Read the model definition and answer for the solid it produces. Units are mm, in the model's axes. A direction names the side the tool comes from. Give positions to 0.01 mm unless a question says otherwise; leave off trailing zeros. Order: outer loops, then holes, each group sorted by start corner. A loop starts at its lowest first (then second) coordinate and runs counter-clockwise, first axis right, second up. Notation, with made-up numbers: M 31.5,33 L 85.5,33 A15 cw 85.5,62 Z; hole C -2.75,63 d3. An arc over 180 degrees is marked long. One line per item, written item: value.
from build123d import *

# Parameters (mm, degrees)
SKETCH1_W           = 12.7
SKETCH1_H           = 50.8
BOSS_EXTRUDE1_DEPTH = 15.113
BOSS_EXTRUDE2_START = 15.113
SKETCH1_3_R         = 25.4
SKETCH1_3_R_2       = 11.303
SKETCH1_3_R_3       = 5.588
SKETCH1_3_W         = 12.7
SKETCH1_3_H         = 50.8
BOSS_EXTRUDE2_DEPTH = 8.636
BOSS_EXTRUDE3_START = 23.749
SKETCH1_4_R         = 5.588
SKETCH1_4_W         = 12.7
SKETCH1_4_H         = 50.8
BOSS_EXTRUDE3_DEPTH = 6.477
SKETCH2_R           = 9.525
CUT_EXTRUDE1_DEPTH  = 130.132211086
SKETCH3_R           = 17.526
CUT_EXTRUDE2_DEPTH  = 2.3876


with BuildPart() as part:
    # Sketch1 → Boss-Extrude1 (new body)
    with BuildSketch(Plane(origin=(0, 0, 0), x_dir=(0, 0, -1), z_dir=(1, 0, 0))):
        with Locations((6.35, 25.4)):
            Rectangle(SKETCH1_W, SKETCH1_H)
    boss_extrude1 = extrude(amount=BOSS_EXTRUDE1_DEPTH)

    # Sketch1_3 → Boss-Extrude2 (add)
    with BuildSketch(Plane(origin=(0, 0, 0), x_dir=(0, 0, -1), z_dir=(1, 0, 0)).offset(BOSS_EXTRUDE2_START)):
        with BuildLine():
            Line((22.86, 50.8), (43.688, 0))
            Line((43.688, 0), (89.408, 0))
            ThreePointArc((89.408, 0), (64.008, 25.4), (89.408, 50.8))
            Line((89.408, 50.8), (22.86, 50.8))
        make_face()
        with Locations((89.408, 25.4)):
            Circle(SKETCH1_3_R)
        with Locations((89.408, 25.4)):
            Circle(SKETCH1_3_R_2, mode=Mode.SUBTRACT)
        Polygon((12.7, 50.8), (12.7, 0), (43.688, 0), (22.86, 50.8), align=None)
        with Locations((28.956, 17.78)):
            Circle(SKETCH1_3_R_3, mode=Mode.SUBTRACT)
        with Locations((6.35, 25.4)):
            Rectangle(SKETCH1_3_W, SKETCH1_3_H)
    boss_extrude2 = extrude(amount=BOSS_EXTRUDE2_DEPTH)

    # Sketch1_4 → Boss-Extrude3 (add)
    with BuildSketch(Plane(origin=(0, 0, 0), x_dir=(0, 0, -1), z_dir=(1, 0, 0)).offset(BOSS_EXTRUDE3_START)):
        Polygon((12.7, 50.8), (12.7, 0), (43.688, 0), (22.86, 50.8), align=None)
        with Locations((28.956, 17.78)):
            Circle(SKETCH1_4_R, mode=Mode.SUBTRACT)
        with Locations((6.35, 25.4)):
            Rectangle(SKETCH1_4_W, SKETCH1_4_H)
    boss_extrude3 = extrude(amount=BOSS_EXTRUDE3_DEPTH)

    # Mirror1: Boss-Extrude1, Boss-Extrude2, Boss-Extrude3 across plane
    add(boss_extrude1.mirror(Plane(origin=(0, 0, 0), x_dir=(0, 0, 1), z_dir=(1, 0, 0))))
    add(boss_extrude2.mirror(Plane(origin=(0, 0, 0), x_dir=(0, 0, 1), z_dir=(1, 0, 0))))
    add(boss_extrude3.mirror(Plane(origin=(0, 0, 0), x_dir=(0, 0, 1), z_dir=(1, 0, 0))))

    # Sketch2 → Cut-Extrude1 (cut, through all)
    with BuildSketch(Plane.XY):
        with Locations((0, 25.4)):
            Circle(SKETCH2_R)
    extrude(amount=-CUT_EXTRUDE1_DEPTH, mode=Mode.SUBTRACT)

    # Sketch3 → Cut-Extrude2 (cut)
    with BuildSketch(Plane.XY):
        with Locations((0, 25.4)):
            Circle(SKETCH3_R)
    extrude(amount=-CUT_EXTRUDE2_DEPTH, mode=Mode.SUBTRACT)


solid = part.part
1) Find section C-C, the plane z = -21. Write down the section's boundary in (x, y).
Reported:
outline: M -30.23,0 L -15.11,0 L -15.11,50.8 L -30.23,50.8 Z; M 15.11,0 L 30.23,0 L 30.23,50.8 L 15.11,50.8 Z
2) Find section D-D, the plane x = 20. Write down the section's boundary in (y, z).
Reported:
outline: M 0,-89.41 A25.4 ccw 50.8,-89.41 L 50.8,0 L 0,0 Z; hole C 17.78,-28.96 d11.18; hole C 25.4,-89.41 d22.61
3) Consider probe 1 along X at (y, z) = (31, -73); probe 2 along Z at (x, y) = (3.5, 3.5); probe 3 along Y at (x, z) = (-19, -84.5). Determine where each line is inside the solid, lowest interval first.
Reported:
probe 1: x = -23.75 to -15.11, 15.11 to 23.75
probe 2: z = -12.7 to 0
probe 3: y = 0 to 15.22, 35.58 to 50.8
4) Determine the mould class of faces 6 (the face through (-19.371, 28.795, -100.189)), 7 (the face through (26.94, 25.04, -33.42)), 8 (the face through (19.371, 28.795, -100.189)), 9 (the face through (21, 0, -34)) for opening direction Z: +Z half, -Z half, draft (parallel to the pull), parting line (faces both ways), or undercut.
Reported:
face 6: undercut
face 7: -Z half
face 8: undercut
face 9: draft
5) Which of the six approach directions +Z, -Z, +X, -X, +Y, -Y give full straight-line access (tool end or side, diameter ignored) to faces 1 (the face through (-23.749, 26, -68)), 2 (the face through (23.749, 26, -68)), 3 (the face through (-3.8, 8.29, -1.18)), 4 (the face through (-2.06, 16.1, -7.47)), 5 (the face through (15.113, 26, -63))?
Reported:
face 1: -Z, -X, +Y
face 2: -Z, +X, +Y
face 3: +Z
face 4: +Z, -Z
face 5: -Z, +Y, -Y
6) Find section B-B, the plane x = 0. Write down the section's boundary in (y, z) (3 decimals), plus the area to 3 significant figures.
Reported:
outline: M 0,-12.7 L 15.875,-12.7 L 15.875,-2.388 L 7.874,-2.388 L 7.874,0 L 0,0 Z; M 34.925,-12.7 L 50.8,-12.7 L 50.8,0 L 42.926,0 L 42.926,-2.388 L 34.925,-2.388 Z
area: 365 mm^2
7) Each of these flat-tipped pins is pushed along its axis until it touches: pin 1 Ø6 at (x, y) = (-23, 13) entering from +Z; pin 2 Ø8 at (y, z) = (21, -40) entering from +X; pin 3 Ø21 at (x, y) = (0, 25.4) entering from +Z; pin 4 Ø15 at (x, y) = (2.5, 34) entering from -Z. Where does it stop, or does it pass through?
Reported:
pin 1: stops at z = 0
pin 2: stops at x = 23.75
pin 3: stops at z = -2.39
pin 4: stops at z = -12.7
8) Find section A-A, the plane y = 25.4. Write down the section's boundary in (x, z) (3 decimals), plus the area to 3 significant figures.
Reported:
outline: M -30.226,-33.274 L -23.749,-33.274 L -23.749,-78.105 L -15.113,-78.105 L -15.113,-12.7 L -9.525,-12.7 L -9.525,-2.388 L -17.526,-2.388 L -17.526,0 L -30.226,0 Z; M -23.749,-114.808 L -15.113,-114.808 L -15.113,-100.711 L -23.749,-100.711 Z; M 9.525,-12.7 L 15.113,-12.7 L 15.113,-78.105 L 23.749,-78.105 L 23.749,-33.274 L 30.226,-33.274 L 30.226,0 L 17.526,0 L 17.526,-2.388 L 9.525,-2.388 Z; M 15.113,-114.808 L 23.749,-114.808 L 23.749,-100.711 L 15.113,-100.711 Z
area: 2,130 mm^2
